Design review of the part built by this model. Coordinates are the model's own, in mm. Coordinates: 2 decimals unless noted, no trailing zeros. Loops run counter-clockwise (first coordinate to the right, second up) from the corner with the lowest first, then second, coordinate; pieces in that order, holes last. Notation, with made-up numbers: (18.5, -2.75) - (67.5, -2.75) arc R15 ccw to (67.5, 12.25) - close; hole circle Ø5 at (18.25, 65). An arc over 180 degrees is marked (long way). Answer in a Markdown table with one row per item. Add a question column.
(1) We need section B-B, the plane z = 0.25. Write out the cut boundary in (x, y), plus the area to 3 significant figures.
(2) We need section A-A, the plane x = 2. Write out the cut boundary in (y, z), plus the area to 3 significant figures.
(3) To check wall thickness, follow L1, parallel to Y at x = -2.75, z = 0.1; L2, parallel to X at y = 0.4, z = 0.2; L3, parallel to Y at x = 7, z = 0.1. State the ranges of each line that lie inside material, in increasing order. Write a range as [from, to].
(4) We need section C-C, the plane x = 10.75. Write out the cut boundary in (y, z).
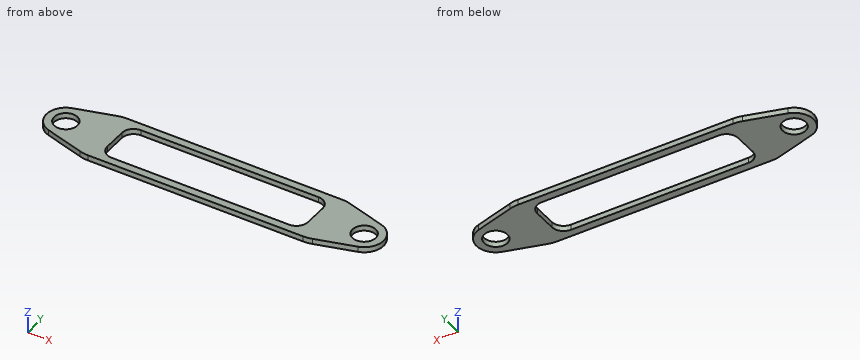
from build123d import *

# Parameters (mm, degrees)
SKETCH1_R           = 0.75
BOSS_EXTRUDE1_DEPTH = 0.35


with BuildPart() as part:
    # Sketch1 → Boss-Extrude1 (new body)
    with BuildSketch(Plane.XY):
        with BuildLine():
            Line((-5.814833275, -1.856361479), (8.113049614, -1.856361479))
            ThreePointArc((8.113049614, -1.856361479), (8.393561593, -1.836592028), (8.668528006, -1.777674508))
            Line((8.668528006, -1.777674508), (11.160598675, -1.057182122))
            ThreePointArc((11.160598675, -1.057182122), (12.06342468, 0.143638521), (11.160598675, 1.344459164))
            Line((11.160598675, 1.344459164), (8.668528006, 2.06495155))
            ThreePointArc((8.668528006, 2.06495155), (8.393561593, 2.123869071), (8.113049614, 2.143638521))
            Line((8.113049614, 2.143638521), (-5.814833275, 2.143638521))
            ThreePointArc((-5.814833275, 2.143638521), (-6.095345255, 2.123869071), (-6.370311667, 2.06495155))
            Line((-6.370311667, 2.06495155), (-8.862382336, 1.344459164))
            ThreePointArc((-8.862382336, 1.344459164), (-9.765208341, 0.143638521), (-8.862382336, -1.057182122))
            Line((-8.862382336, -1.057182122), (-6.370311667, -1.777674508))
            ThreePointArc((-6.370311667, -1.777674508), (-6.095345255, -1.836592028), (-5.814833275, -1.856361479))
        make_face()
        with Locations((-8.515208341, 0.143638521)):
            Circle(SKETCH1_R, mode=Mode.SUBTRACT)
        with Locations((10.81342468, 0.143638521)):
            Circle(SKETCH1_R, mode=Mode.SUBTRACT)
        with BuildLine():
            Line((7.649108169, -0.606361479), (7.649108169, 0.893638521))
            ThreePointArc((7.649108169, 0.893638521), (7.429438255, 1.423968607), (6.899108169, 1.643638521))
            Line((6.899108169, 1.643638521), (-4.600891831, 1.643638521))
            ThreePointArc((-4.600891831, 1.643638521), (-5.131221917, 1.423968607), (-5.350891831, 0.893638521))
            Line((-5.350891831, 0.893638521), (-5.350891831, -0.606361479))
            ThreePointArc((-5.350891831, -0.606361479), (-5.131221917, -1.136691565), (-4.600891831, -1.356361479))
            Line((-4.600891831, -1.356361479), (6.899108169, -1.356361479))
            ThreePointArc((6.899108169, -1.356361479), (7.429438255, -1.136691565), (7.649108169, -0.606361479))
        make_face(mode=Mode.SUBTRACT)
    extrude(amount=BOSS_EXTRUDE1_DEPTH)


solid = part.part
Responses:
| question | item | result |
|---|---|---|
| 1 | outline | (-8.86, -1.06) - (-6.37, -1.78) arc R2 ccw to (-5.81, -1.86) - (8.11, -1.86) arc R2 ccw to (8.67, -1.78) - (11.16, -1.06) arc R1.25 ccw to (11.16, 1.34) - (8.67, 2.06) arc R2 ccw to (8.11, 2.14) - (-5.81, 2.14) arc R2 ccw to (-6.37, 2.06) - (-8.86, 1.34) arc R1.25 ccw to start; hole circle Ø1.5 at (-8.52, 0.14); hole (-5.35, -0.61) arc R0.75 ccw to (-4.6, -1.36) - (6.9, -1.36) arc R0.75 ccw to (7.65, -0.61) - (7.65, 0.89) arc R0.75 ccw to (6.9, 1.64) - (-4.6, 1.64) arc R0.75 ccw to (-5.35, 0.89) - close; hole circle Ø1.5 at (10.81, 0.14) |
| 1 | area | 36.8 mm2 |
| 2 | outline | (-1.86, 0) - (-1.36, 0) - (-1.36, 0.35) - (-1.86, 0.35) - close; (1.64, 0) - (2.14, 0) - (2.14, 0.35) - (1.64, 0.35) - close |
| 2 | area | 0.350 mm2 |
| 3 | L1 | y = [-1.86, -1.36], [1.64, 2.14] |
| 3 | L2 | x = [-9.74, -9.22], [-7.81, -5.35], [7.65, 10.11], [11.52, 12.04] |
| 3 | L3 | y = [-1.86, -1.35], [1.64, 2.14] |
| 4 | outline | (-1.18, 0) - (-0.6, 0) - (-0.6, 0.35) - (-1.18, 0.35) - close; (0.89, 0) - (1.46, 0) - (1.46, 0.35) - (0.89, 0.35) - close |
